Autodesk Inventor part; units mm, degrees
ref_plane "YZ Plane" through (0, 0, 0) normal (1, 0, 0) x (0, 1, 0)
ref_plane "XZ Plane" through (0, 0, 0) normal (0, 1, 0) x (-1, 0, 0)
ref_plane "XY Plane" through (0, 0, 0) normal (0, 0, 1) x (1, 0, 0)
sketch "Sketch1" plane through (0, 0, 0) normal (0, 1, 0) x (-1, 0, 0)
  line L0 (10, -15.715) -> (-10, -15.715)
  line L1 (-10, -15.715) -> (-10, 15.715)
  line L2 (-10, 15.715) -> (10, 15.715)
  line L3 (10, 15.715) -> (10, -15.715)
  point P0 (0, 0)
  dimension "d0" = 20
  dimension "d1" = 31.43
  dimension "d2" = 10
  dimension "d3" = 15.715
extrude "Plate1" add sketch "Sketch1" along normal blind 1.5
sketch "Sketch2" plane through (10, 0, 17.215) normal (0, 0, -1) x (-1, 0, 0)
  line L0 (20, 0) -> (0, 0)
  line L1 (0, 0) -> (0, 40)
  line L2 (0, 40) -> (20, 40)
  line L3 (20, 40) -> (20, 0)
edge flange "Flange1" height 40 angle 90 thickness 1.5 bend radius 0.31 thickness toward (0, 0, -1) relief tear relief width 1.5 relief depth 0.75 edges at (0, 1.5, 15.715) wall of the first edge with corners at (-10, 0, 17.215) (10, 0, 17.215) (10, 40, 17.215) (-10, 40, 17.215)
bend "Bend1"
corner "Corner1"
sketch "Sketch3" plane through (-10, 0, -17.215) normal (0, 0, 1) x (1, 0, 0)
  line L0 (20, 0) -> (0, 0)
  line L1 (0, 0) -> (0, 40)
  line L2 (0, 40) -> (20, 40)
  line L3 (20, 40) -> (20, 0)
edge flange "Flange2" height 40 angle 90 thickness 1.5 bend radius 0.31 thickness toward (0, 0, 1) relief tear relief width 1.5 relief depth 0.75 edges at (0, 1.5, -15.715) wall of the first edge with corners at (10, 0, -17.215) (-10, 0, -17.215) (-10, 40, -17.215) (10, 40, -17.215)
bend "Bend2"
corner "Corner2"
sketch "Sketch4" plane through (10, 40, 15.715) normal (0, 0, -1) x (-1, 0, 0)
  line L0 (30.46, -23.2265) -> (30.46, -24.7935)
  line L1 (38.57, -15.71) -> (38.57, -17.31)
  circle A0 centre (3, -16.51) radius 0.7835
  circle A1 centre (10, -9.51) radius 0.7835
  line L2 (38.57, -15.71) -> (38.57, -17.31)
  line L3 (38.57, -15.71) -> (38.57, -17.31)
  line L4 (37.07, -17.31) -> (37.07, -15.71)
  line L5 (30.46, -23.2265) -> (30.46, -24.7935)
  circle A2 centre (10, -23.51) radius 0.7835
  circle A3 centre (3, -16.51) radius 0.7835
  circle A4 centre (17, -16.51) radius 0.7835
  circle A5 centre (10, -9.51) radius 0.7835
  point P0 (10, -40)
hole "Hole1" at (0, 16.49, 15.715) at (-7, 23.49, 15.715) at (0, 30.49, 15.715) at (7, 23.49, 15.715) direction (0, 0, 1) diameter 1.6 depth 1.5
sketch "Sketch5" plane through (0, 1.5, 0) normal (0, 1, 0) x (1, 0, 0)
  circle A0 centre (-7, -2.785) radius 0.7835
  circle A1 centre (0, -9.785) radius 0.7835
  circle A2 centre (7, -2.785) radius 0.7835
  circle A3 centre (0, 4.215) radius 0.7835
  point P0 (0, 0)
hole "Hole2" at (-7, 1.5, 2.785) at (0, 1.5, 9.785) at (7, 1.5, 2.785) at (0, 1.5, -4.215) direction (0, -1, 0) diameter 1.6 depth 1.5
equation "\"d30\" = Thickness"
equation "\"d37\" = Thickness"
equation "\"d4\" = Thickness"
equation "\"d5\" = BendReliefWidth"
equation "\"d6\" = BendReliefDepth"
equation "\"d7\" = MinimumRemnant"
equation "\"d8\" = TransitionRadius"
equation "\"d11\" = BendRadius"
equation "\"d12\" = CornerReliefSize"
equation "\"d13\" = GapSize"
equation "\"d14\" = JacobiRadiusSize"
equation "\"d15\" = BendReliefWidth"
equation "\"d16\" = BendReliefDepth"
equation "\"d17\" = MinimumRemnant"
equation "\"d18\" = TransitionRadius"
equation "\"d21\" = BendRadius"
equation "\"d22\" = CornerReliefSize"
equation "\"d23\" = GapSize"
equation "\"d24\" = JacobiRadiusSize"
equation "\"BendReliefWidth\" = Thickness"
equation "\"BendReliefDepth\" = 0.5 * Thickness"
equation "\"CornerReliefSize\" = 4 * Thickness"
equation "\"MinimumRemnant\" = 2 * Thickness"
equation "\"TransitionRadius\" = BendRadius"
equation "\"JacobiRadiusSize\" = BendRadius"
equation "\"GapSize\" = Thickness"
properties part number "axis_7_top_frame" material "Aluminum 6061-AHC"
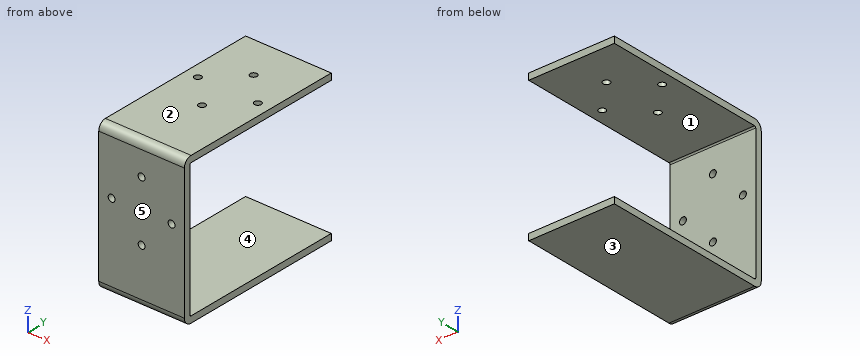
Model file for the job. Use its own axes, mm. Face numbers are marked on the shaded views. A direction names the side the tool comes from. Give positions to 0.01 mm unless a question says otherwise; leave off trailing zeros. Loops run counter-clockwise (first coordinate to the right, second up) from the corner with the lowest first, then second, coordinate; pieces in that order, holes last. Notation, with made-up numbers: (88.5, 59) -> (99.5, 59) arc R24 ccw to (99.5, 70) -> close; hole circle Ø9 at (46, -35). An arc over 180 degrees is marked (long way). Use a Markdown table: item, result. Add a question column.
(1) Tool access for the marked faces 4 and 5: list every direction of +Z, -Z, +X, -X, +Y, -Y with a clear straight run to the whole face (end or side of a thin tool).
(2) Slice it at C-C on y = 25.5. List the corners of the cut face in (x, z) (3 decimals).
(3) Slice it at B-B on x = 0. List the corners of the cut face in (y, z) (3 decimals), and give its area (3 significant figures).
(4) Slice it at D-D on z = 10. List the corners of the cut face in (x, y).
(5) Mould opens along Z. For the marked faces 1, 2 and 3 say: +Z half, -Z half, draft (parallel to the pull), parting line (faces both ways), or undercut.
(6) Wall check: line 1 along Z through (x, y) = (-6.75, 6.5) (3 decimals); line 2 along X through (y, z) = (23.49, 16.65); line 3 along Z through (x, y) = (0, 0.65) (3 decimals). Give the ranges that are in metal, low to high.
(7) Drop flat-ended pins along their axis: pin 1 Ø1.8 at (x, z) = (0, 9.785) entering from +Y; pin 2 Ø1 at (x, z) = (7, 2.785) entering from +Y. Give the stop position or say it passes through.
(8) Slice it at A-A on y = 16.49. List the corners of the cut face in (x, z) (3 decimals).
Filled sheet:
| question | item | result |
|---|---|---|
| 1 | face 4 | +X, -X, +Y |
| 1 | face 5 | +Z, -Z, +X, -X, -Y |
| 2 | outline | (-10, -17.215) -> (10, -17.215) -> (10, -15.715) -> (-10, -15.715) -> close; (-10, 15.715) -> (10, 15.715) -> (10, 17.215) -> (-10, 17.215) -> close |
| 3 | outline | (0, -15.405) arc R1.81 ccw to (1.81, -17.215) -> (40, -17.215) -> (40, -15.715) -> (1.81, -15.715) arc R0.31 cw to (1.5, -15.405) -> (1.5, -5.015) -> (0, -5.015) -> close; (0, -3.415) -> (1.5, -3.415) -> (1.5, 8.985) -> (0, 8.985) -> close; (0, 10.585) -> (1.5, 10.585) -> (1.5, 15.405) arc R0.31 cw to (1.81, 15.715) -> (15.69, 15.715) -> (15.69, 17.215) -> (1.81, 17.215) arc R1.81 ccw to (0, 15.405) -> close; (17.29, 15.715) -> (29.69, 15.715) -> (29.69, 17.215) -> (17.29, 17.215) -> close; (31.29, 15.715) -> (40, 15.715) -> (40, 17.215) -> (31.29, 17.215) -> close |
| 3 | area | 156 mm2 |
| 4 | outline | (-10, 0) -> (-0.77, 0) -> (-0.77, 1.5) -> (-10, 1.5) -> close; (0.77, 0) -> (10, 0) -> (10, 1.5) -> (0.77, 1.5) -> close |
| 5 | face 1 | undercut |
| 5 | face 2 | +Z half |
| 5 | face 3 | -Z half |
| 6 | line 1 | -17.215 to -15.715, 15.715 to 17.215 |
| 6 | line 2 | -10 to -7.8, -6.2 to 6.2, 7.8 to 10 |
| 6 | line 3 | -16.794 to -5.015, -3.415 to 8.985, 10.585 to 16.794 |
| 7 | pin 1 | y = 1.5 |
| 7 | pin 2 | through |
| 8 | outline | (-10, -17.215) -> (10, -17.215) -> (10, -15.715) -> (-10, -15.715) -> close; (-10, 15.715) -> (-0.8, 15.715) -> (-0.8, 17.215) -> (-10, 17.215) -> close; (0.8, 15.715) -> (10, 15.715) -> (10, 17.215) -> (0.8, 17.215) -> close |
